Here's how the part is built. I have some questions about the finished solid (model axes, mm). A direction names the side the tool comes from. Give positions to 0.01 mm unless a question says otherwise; leave off trailing zeros. Write each loop counter-clockwise with the first axis right and the second up, starting at its lowest first coordinate (ties: lowest second). Pieces come first, ordered by that corner, then holes. Notation, with made-up numbers: M 63.25,-13 L 76.25,-13 A20 cw 76.25,-1 Z; hole C -32,76.5 d3. An arc over 180 degrees is marked long. Answer as CSV lines item,"result". Start each with the question number.
Q1. Suppose I cut it at B-B (y = -5.5). Write out the boundary of the cut face in (x, z).
Q2. If I drill on line 1 along Y through (x, z) = (3.25, 0); line 2 along Z through (x, y) = (2.9, -8); line 3 along Z through (x, y) = (0.9, 8.5), over which ranges is the centre line in solid material (lowest first)?
Q3. Suppose I cut it at A-A (x = 0.7). Count the separate pieces of the cut face and the enclosed holes in it, then the cut area to 3 significant figures.
Q4. Suppose I cut it at C-C (y = -1.5). Write out the boundary of the cut face in (x, z), then the cut area to 3 significant figures.
Q5. For pin 1 (5 mm diameter, centred on y = -3.5, z = 7, fed in from -X); pin 2 (1.1 mm diameter, centred on y = 0, z = 0, fed in from +X); pin 3 (1 mm diameter, centred on x = 3, z = -6, fed in from +Y); pin 4 (2.5 mm diameter, centred on y = 0.5, z = 1, fed in from +X), each with a flat end and sliding along its axis, tell me the tip position at first contact or that it passes through.
Q6. On a 3-axis mill with a long thin cutter (end or side, diameter ignored), from which of +Z, -Z, +X, -X, +Y, -Y can I reach the whole of each face in a straight line? I mean faces 4 (the cylindrical face through (2.07, -5.09, 7.06)), 5 (the cylindrical face through (2.071, -4.2, 7.595)), 6 (the flat face through (2.6, -0.5, -1)), 7 (the cylindrical face through (2.07, 1.11, -8.61)), 8 (the cylindrical face through (2.071, -8.522, -1.648)). Say none if no direction works.
Q7. Thinking about a two-plate mould opening in Z: for faces 1 (the flat face through (0, -6, -3)), 2 (the cylindrical face through (2.07, 1.12, 8.63)), 3 (the cylindrical face through (2.071, 8.248, 2.703)), which applies, +Z half, -Z half, draft (parallel to the pull), parting line (faces both ways), or undercut?
```python
from build123d import *

# Parameters (mm, degrees)
BASPROSKE_W         = 4.2
BASPROSKE_H         = 9.45
TOOTHCUT_DEPTH      = 15.008747267
TEETHCUTS_COUNT     = 25
TEETHCUTS_ANGLE     = 345.6
SKETCH7_R           = 2.4
CUT_EXTRUDE2_DEPTH  = 1.6
SKETCH13_R          = 6.5
SKETCH13_R_2        = 3
CUT_EXTRUDE3_DEPTH  = 1.2
CUT_EXTRUDE4_START  = -1.2
SKETCH15_R          = 6.5
SKETCH15_R_2        = 3
CUT_EXTRUDE4_DEPTH  = 1.2
CUT_EXTRUDE5_START  = -1.6
SKETCH17_R          = 2.4
CUT_EXTRUDE5_DEPTH  = 1.6
SKETCH18_R          = 0.9
CUT_EXTRUDE6_DEPTH  = 1.6
SKETCH19_R          = 3
SKETCH19_R_2        = 2.4
BOSS_EXTRUDE1_DEPTH = 0.6


with BuildPart() as part:
    # BasProSke → Base-Revolve (revolve)
    with BuildSketch(Plane(origin=(0, 0, 0), x_dir=(1, 0, 0), z_dir=(0, 1, 0)), mode=Mode.PRIVATE) as base_revolve_sk:
        with Locations((2.1, 4.725)):
            Rectangle(BASPROSKE_W, BASPROSKE_H)
    revolve(base_revolve_sk.sketch.rotate(Axis((-10, 0, 0), (1, 0, 0)), 180), axis=Axis((-10, 0, 0), (1, 0, 0)))

    # TooCutSke → ToothCut (cut, through all)
    with BuildSketch(Plane(origin=(0, 0, 0), x_dir=(0, 0, -1), z_dir=(1, 0, 0))):
        with BuildLine():
            ThreePointArc((0.336642775, 7.866800343), (0, 7.874), (-0.336642775, 7.866800343))
            ThreePointArc((-0.336642775, 7.866800343), (-0.577188207, 8.685445672), (-1.008672355, 9.421559597))
            ThreePointArc((-1.008672355, 9.421559597), (0, 9.4754), (1.008672355, 9.421559597))
            ThreePointArc((1.008672355, 9.421559597), (0.577188207, 8.685445672), (0.336642775, 7.866800343))
        make_face()
    toothcut = extrude(amount=TOOTHCUT_DEPTH, mode=Mode.SUBTRACT)

    # TeethCuts: ToothCut ×25 about axis
    teethcuts_axis = Axis((-10, 0, 0), (1, 0, 0))
    for i in range(1, TEETHCUTS_COUNT):
        add(toothcut.rotate(teethcuts_axis, i * TEETHCUTS_ANGLE / (TEETHCUTS_COUNT - 1)), mode=Mode.SUBTRACT)

    # Sketch7 → Cut-Extrude2 (cut)
    with BuildSketch(Plane(origin=(4.2, 0, 0), x_dir=(0, 0, -1), z_dir=(1, 0, 0))):
        Circle(SKETCH7_R)
    extrude(amount=-CUT_EXTRUDE2_DEPTH, mode=Mode.SUBTRACT)

    # Sketch13 → Cut-Extrude3 (cut)
    with BuildSketch(Plane(origin=(4.2, 0, 0), x_dir=(0, 0, -1), z_dir=(1, 0, 0))):
        Circle(SKETCH13_R)
        Circle(SKETCH13_R_2, mode=Mode.SUBTRACT)
    extrude(amount=-CUT_EXTRUDE3_DEPTH, mode=Mode.SUBTRACT)

    # Sketch15 → Cut-Extrude4 (cut)
    with BuildSketch(Plane.ZY.offset(CUT_EXTRUDE4_START)):
        with Locations(Location((0, 0, 0), (0, 0, 180))):
            Circle(SKETCH15_R)
        with Locations(Location((0, 0, 0), (0, 0, 180))):
            Circle(SKETCH15_R_2, mode=Mode.SUBTRACT)
    extrude(amount=CUT_EXTRUDE4_DEPTH, mode=Mode.SUBTRACT)

    # Sketch17 → Cut-Extrude5 (cut)
    with BuildSketch(Plane.ZY.offset(CUT_EXTRUDE5_START)):
        with Locations(Location((0, 0, 0), (0, 0, 180))):
            Circle(SKETCH17_R)
    extrude(amount=CUT_EXTRUDE5_DEPTH, mode=Mode.SUBTRACT)

    # Sketch18 → Cut-Extrude6 (cut)
    with BuildSketch(Plane(origin=(2.6, 0, 0), x_dir=(0, 0, -1), z_dir=(1, 0, 0))):
        Circle(SKETCH18_R)
    extrude(amount=-CUT_EXTRUDE6_DEPTH, mode=Mode.SUBTRACT)

    # Sketch19 → Boss-Extrude1 (add)
    with BuildSketch(Plane.ZY):
        with Locations(Location((0, 0, 0), (0, 0, 180))):
            Circle(SKETCH19_R)
        with Locations(Location((0, 0, 0), (0, 0, 180))):
            Circle(SKETCH19_R_2, mode=Mode.SUBTRACT)
    extrude(amount=BOSS_EXTRUDE1_DEPTH)


solid = part.part
```
Resolved:
1,outline,"M 0,-6.03 L 4.2,-6.03 L 4.2,-3.46 L 3,-3.46 L 3,3.46 L 4.2,3.46 L 4.2,6.03 L 0,6.03 L 0,3.46 L 1.2,3.46 L 1.2,-3.46 L 0,-3.46 Z"
2,line 1,"-9.45 to -6.5, -3 to -2.4, 2.4 to 3, 6.5 to 7.87"
2,line 2,"-4.72 to -3.88, -2.66 to -1.4, -0.64 to 0.64, 1.4 to 2.66, 3.88 to 4.72"
2,line 3,"-3.68 to -2.91, -1.61 to -0.5, 0.5 to 1.61, 2.91 to 3.68"
3,separate pieces,"2"
3,enclosed holes,"2"
3,area,"111 mm^2"
4,outline,"M -0.6,-2.6 L 1.2,-2.6 L 1.2,-6.32 L 0,-6.32 L 0,-7.73 L 4.2,-7.73 L 4.2,-6.32 L 3,-6.32 L 3,-2.6 L 4.2,-2.6 L 4.2,-1.87 L 2.6,-1.87 L 2.6,1.87 L 4.2,1.87 L 4.2,2.6 L 3,2.6 L 3,6.32 L 4.2,6.32 L 4.2,7.73 L 0,7.73 L 0,6.32 L 1.2,6.32 L 1.2,2.6 L -0.6,2.6 L -0.6,1.87 L 1.6,1.87 L 1.6,-1.87 L -0.6,-1.87 Z"
4,area,"35.9 mm^2"
5,pin 1,"x = 0"
5,pin 2,"through"
5,pin 3,"y = 7.68"
5,pin 4,"x = 2.6"
6,face 4,"+X, -X"
6,face 5,"+Z, +X, -X"
6,face 6,"+X"
6,face 7,"-Z, +X, -X"
6,face 8,"+X, -X, -Y"
7,face 1,"draft"
7,face 2,"+Z half"
7,face 3,"undercut"
